from build123d import *

# Parameters (mm, degrees)
F3_DEPTH = 22.225
F4_R     = 1.27


with BuildPart() as f1:
    # F0 (on Front) → F1 (revolve)
    with BuildSketch(Plane.XZ):
        Polygon((41.9079282205, 22.225), (40.6379282205, 0), (41.91, 0), (43.18, 22.225), align=None)
    revolve(axis=Axis((0, 0, 4.1103595868), (0, 0, 1)))

    # F2 (on Top) → F3 (join, through all)
    with BuildSketch(Plane.XY):
        with BuildLine():
            ThreePointArc((0.635, 41.9051891178), (0, 41.91), (-0.635, 41.9051891178))
            Line((-0.635, 41.9051891178), (-0.635, -41.9051891178))
            ThreePointArc((-0.635, -41.9051891178), (0, -41.91), (0.635, -41.9051891178))
            Line((0.635, -41.9051891178), (0.635, 41.9051891178))
        make_face()
    extrude(amount=F3_DEPTH)

    # F4
    f4_edges = [f1.edges().sort_by_distance(p)[0] for p in [
        (0.635, -41.268043, 11.1125),
        (0.635, 41.268043, 11.1125),
        (-0.635, 41.268043, 11.1125),
        (-0.635, -41.268043, 11.1125),
    ]]
    fillet(f4_edges, radius=F4_R)


solid = f1.part
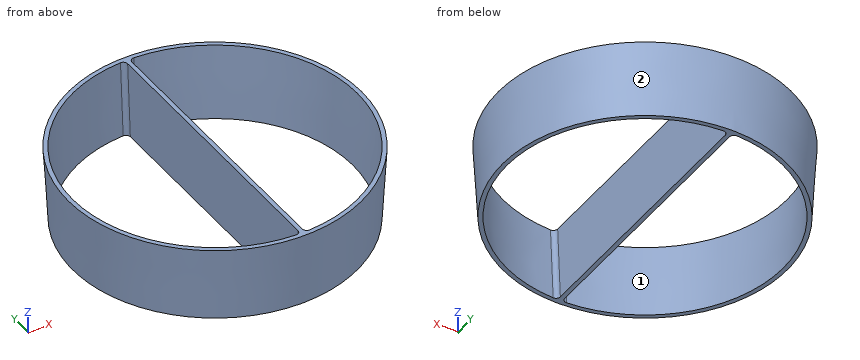
CAD build for the part. Positions are in the model's coordinates, mm. Face numbers are marked on the shaded views. Round coordinates to 2 decimals unless told otherwise and drop trailing zeros.
(1) Two-plate mould, pull along X, no slides. Class the marked faces 1 and 2: +X half, -X half, draft (parallel to the pull), parting line (faces both ways), or undercut.
(2) Drop flat-ended pins along their axis: pin 1 (10 mm diameter, centred on x = -28.5, z = 6.5, fed in from -Y); pin 2 (1.5 mm diameter, centred on x = -32, y = -23.5, fed in from +Z); pin 3 (3 mm diameter, centred on x = 19.5, z = 13.5, fed in from +Y); pin 4 (10 mm diameter, centred on y = -26.5, z = 15, fed in from -X). Give the stop position or say it passes through.
(3) Wall check: line 1 along X through (y, z) = (-1, 19.5) (3 decimals); line 2 along X through (y, z) = (-27, 8) (3 decimals); line 3 along Y through (x, z) = (26, 6.5). Give the ranges that are in metal, low to high.
(4) Cut at B-B (z = 4). State how many separate pieces and enclosed holes the cut face has, plus the area to 3 significant figures.
Findings below:
1. face 1: undercut
1. face 2: parting line
2. pin 1: stops at y = -35.17
2. pin 2: passes through
2. pin 3: stops at y = 38.71
2. pin 4: stops at x = -36.99
3. line 1: x = -43.013 to -41.74, -0.635 to 0.635, 41.74 to 43.013
3. line 2: x = -32.649 to -30.981, -0.635 to 0.635, 30.981 to 32.649
3. line 3: y = -33.34 to -31.71, 31.71 to 33.34
4. separate pieces: 1
4. enclosed holes: 2
4. area: 437 mm2
